Read the model definition and answer for the solid it produces. Units are mm, in the model's axes. A direction names the side the tool comes from. Coordinates: 2 decimals unless noted, no trailing zeros. Write each loop counter-clockwise with the first axis right and the second up, starting at its lowest first coordinate (ties: lowest second). Pieces come first, ordered by that corner, then holes.
(1) The part is cut by section D-D, the plane z = 6.5. Determine the outline of the cut face in (x, y).
(2) Straight lines are drawn through the part: line 1 along Y through (x, z) = (-20, 63); line 2 along X through (y, z) = (0.5, 18.5); line 3 along X through (y, z) = (4.75, 13). For each, find the intervals that lie inside material, in ascending order.
(3) The part is cut by section B-B, the plane z = 15.5. Determine the outline of the cut face in (x, y), and give its area (3 significant figures).
(4) Determine the mould class of faces 4 (the cylindrical face through (19.232, -1.542, 64.785)), 5 (the cylindrical face through (-11.507, -4.03, 41.532)), 6 (the flat face through (-20, -14.3, 37.2)) for opening direction X: pulls with the +X half, pulls with the -X half, needs draft (parallel to the pull), parting line crosses it, or undercut.
(5) Given pin 1 (11 mm diameter, centred on x = 0, z = 13, fed in from -Y); pin 2 (1 mm diameter, centred on x = 11.5, z = 50, fed in from -Y); pin 3 (5 mm diameter, centred on x = -3.5, z = 36, fed in from -Y), each flat-ended and moving along its own axis, determine where each tip first touches the part or whether it passes through.
(6) The part is cut by section A-A, the plane y = 10. State how many separate pieces and enclosed holes the cut face has, and give its area (3 significant figures).
(7) Which of the six approach directions +Z, -Z, +X, -X, +Y, -Y give full straight-line access (tool end or side, diameter ignored) to faces 1 (the flat face through (20, -14.3, 37)), 2 (the flat face through (-20, 20, 41)), 3 (the flat face through (-0.203, 6.789, 36.815))?
```python
from build123d import *

# Parameters (mm, degrees)
F0_R      = 12.9
F1_DEPTH  = 28
F2_W      = 45
F2_H      = 45
F3_DEPTH  = 50
F5_DEPTH  = 45.001
F6_R      = 14.5
F7_DEPTH  = 35
F8_R      = 16.1
F9_DEPTH  = 20
F10_R     = 3.4
F11_DEPTH = 32.8
F12_R     = 1.2
F12_R_2   = 7
F13_DEPTH = 65.2
F15_DEPTH = 45.0010001
F16_R     = 1.2
F17_DEPTH = 46.3874578725
F18_SIZE  = 5
F19_SIZE  = 1


with BuildPart() as f1:
    # F0 (on Top) → F1 (new body)
    with BuildSketch(Plane.XY):
        Circle(F0_R)
    extrude(amount=F1_DEPTH)

    # F2 (on face) → F3 (join)
    with BuildSketch(Plane.XY.offset(28)):
        Rectangle(F2_W, F2_H)
    extrude(amount=F3_DEPTH)

    # F4 (on face) → F5 (cut, through all)
    with BuildSketch(Plane.YZ.offset(22.5)):
        Polygon((-22.5, 78), (-22.5, 64.6205767989), (22.5, 78), align=None)
    extrude(amount=-F5_DEPTH, mode=Mode.SUBTRACT)

    # F6 (on face) → F7 (cut)
    with BuildSketch(Plane(origin=(0, -19.4799905068, 65.5184875785), x_dir=(1, 0, 0), z_dir=(0, -0.2849907161, 0.9585302769))):
        with Locations((0, 16.7962070879)):
            Circle(F6_R)
    extrude(amount=-F7_DEPTH, mode=Mode.SUBTRACT)

    # F8 (on face) → F9 (cut)
    with BuildSketch(Plane(origin=(0, -19.4799905068, 65.5184875785), x_dir=(1, 0, 0), z_dir=(0, -0.2849907161, 0.9585302769))):
        with Locations((0, 16.7962070879)):
            Circle(F8_R)
    extrude(amount=-F9_DEPTH, mode=Mode.SUBTRACT)

    # F10 (on Front) → F11 (cut, symmetric)
    with BuildSketch(Plane.XZ):
        with Locations((0, 13)):
            Circle(F10_R)
    extrude(amount=F11_DEPTH, both=True, mode=Mode.SUBTRACT)

    # F12 (on Right) → F13 (cut, symmetric)
    with BuildSketch(Plane.YZ):
        with Locations((-1.3853824633, 63.5955387264)):
            Circle(F12_R)
        with Locations((4.3748263706, 44.2218038779)):
            Circle(F12_R_2)
    extrude(amount=F13_DEPTH, both=True, mode=Mode.SUBTRACT)

    # F14 (on face) → F15 (cut, through all)
    with BuildSketch(Plane.YZ.offset(22.5)):
        Polygon((-16.8001856775, 45.449971261), (-22.5, 64.6205767989), (-22.5, 43.755299528), align=None)
        Polygon((-16.8001856775, 28), (-16.8001856775, 45.449971261), (-22.5, 43.755299528), (-22.5, 28), align=None)
        Polygon((22.5, 78), (15.8861410894, 76.0335640587), (22.5, 53.7886850006), align=None)
    extrude(amount=-F15_DEPTH, mode=Mode.SUBTRACT)

    # F16 (on face) → F17 (cut, through all)
    with BuildSketch(Plane(origin=(0, -3.0200094932, -0.8979107796), x_dir=(1, 0, 0), z_dir=(0, -0.9585302769, -0.2849907161))):
        with Locations((0, 61.3530704849)):
            Circle(F16_R)
    extrude(amount=-F17_DEPTH, mode=Mode.SUBTRACT)

    # F18
    f18_edges = [f1.edges().sort_by_distance(p)[0] for p in [
        (22.5, -19.650093, 55.035274),
        (22.5, -16.800186, 36.724986),
        (22.5, 19.193071, 64.911125),
        (22.5, 22.5, 40.894343),
        (-22.5, 22.5, 40.894343),
        (-22.5, 19.193071, 64.911125),
        (-22.5, -19.650093, 55.035274),
        (-22.5, -16.800186, 36.724986),
        (-12.9, 0, 0),
    ]]
    chamfer(f18_edges, length=F18_SIZE)

    # F19
    f19_edges = [f1.edges().sort_by_distance(p)[0] for p in [
        (-16.1, -3.380317, 70.305251),
        (22.5, -2.625174, 44.221804),
        (-22.5, -2.625174, 44.221804),
    ]]
    chamfer(f19_edges, length=F19_SIZE)


solid = f1.part
```
Computed:
1. outline: circle Ø25.8 at (0, 0)
2. line 1: y = -19.41 to -2.43, -0.34 to 17.15
2. line 2: x = -12.89 to 12.89
2. line 3: x = -11.99 to -3.4, 3.4 to 11.99
3. outline: (-2.3, -12.69) - (-2.3, 12.69) arc R12.9 ccw to start; (2.3, -12.69) arc R12.9 ccw to (2.3, 12.69) - close
3. area: 405 mm2
4. face 4: needs draft
4. face 5: undercut
4. face 6: pulls with the -X half
5. pin 1: stops at y = -12.9
5. pin 2: stops at y = -18.3
5. pin 3: stops at y = -16.8
6. separate pieces: 3
6. enclosed holes: 1
6. area: 1,400 mm2
7. face 1: -Z, +X, -Y
7. face 2: +Z, -Z, -X, +Y
7. face 3: none
